```python
from build123d import *

# Parameters (mm, degrees)
SKETCH_W     = 15.4
SKETCH_H     = 6.2
SKETCH_R     = 1.6
PAD_DEPTH    = 6.2
SKETCH001_R  = 1.6
POCKET_DEPTH = 6.201
FILLET_R     = 3
FILLET001_R  = 3


with BuildPart() as part:
    # Sketch → Pad (new body)
    with BuildSketch(Plane.XY):
        with Locations((4.6, 0)):
            Rectangle(SKETCH_W, SKETCH_H)
        Circle(SKETCH_R, mode=Mode.SUBTRACT)
    extrude(amount=PAD_DEPTH)

    # Sketch001 (on Face1 of Pad) → Pocket (cut, through all)
    with BuildSketch(Plane(origin=(0, 3.1, 0), x_dir=(-1, 0, 0), z_dir=(0, 1, 0))):
        with Locations((-9.2, 3.1)):
            Circle(SKETCH001_R)
    extrude(amount=-POCKET_DEPTH, mode=Mode.SUBTRACT)

    # Fillet
    fillet_edges = [part.edges().sort_by_distance(p)[0] for p in [
        (-3.1, -3.1, 3.1),
        (-3.1, 3.1, 3.1),
    ]]
    fillet(fillet_edges, radius=FILLET_R)

    # Fillet001
    fillet001_edges = [part.edges().sort_by_distance(p)[0] for p in [
        (12.3, 0, 6.2),
        (12.3, 0, 0),
    ]]
    fillet(fillet001_edges, radius=FILLET001_R)


solid = part.part
```
CAD build for the part. Positions are in the model's coordinates, mm. Coordinates: 2 decimals unless noted, no trailing zeros. Order: outer loops, then holes, each group sorted by start corner. A loop starts at its lowest first (then second) coordinate and runs counter-clockwise, first axis right, second up. Notation, with made-up numbers: (34, 79) -> (64, 79) arc R14 ccw to (64, 89) -> close; hole circle Ø2 at (32, 69). An arc over 180 degrees is marked (long way). Use one line per item in the form item = value. Start each with the question number.
1) Pull direction Y, two halves, no side cores. Call faces 1 (the cylindrical face through (-2.24, -2.2, 3.14)), 2 (the cylindrical face through (-1.27, -0.97, 3.06)), 3 (the flat face through (4, 0, 6.2)), 4 (the cylindrical face through (-2.24, 2.2, 3.14)): +Y half, -Y half, draft (parallel to the pull), parting line (faces both ways), or undercut.
2) Drill centre lines: L1, parallel to X at y = 0.5, z = 2.25; L2, parallel to Z at x = 9.2, y = 1.5; L3, parallel to X at y = 0.5, z = 4.25. Where is each one in solid material? Low to high. Write a range as [from, to].
3) Drop a flat-ended pin along its axis: pin 1 (2 mm diameter, centred on y = -1, z = 5, fed in from -X). Give the stop position or say it passes through.
4) Band-saw the part on B-B on z = 2.75. Give the cut face in (x, y), then the cut area to 3 significant figures.
5) Band-saw the part on D-D on z = 5.75. Give the cut face in (x, y), then the cut area to 3 significant figures.
6) Band-saw the part on A-A on y = 1.25. Give the cut face in (x, z).
7) Band-saw the part on C-C on x = 0.25. Give the cut face in (y, z), then the cut area to 3 significant figures.
Entries:
q1.face_1 = -Y half
q1.face_2 = undercut
q1.face_3 = draft
q1.face_4 = +Y half
q2.L1 = [-3.07, -1.52], [1.52, 7.84], [10.56, 12.2]
q2.L2 = [0, 1.5], [4.7, 6.2]
q2.L3 = [-3.07, -1.52], [1.52, 8.09], [10.31, 12.11]
q3.pin_1 = -3.1
q4.outline = (-3.1, -0.1) arc R3 ccw to (-0.1, -3.1) -> (7.64, -3.1) -> (7.64, 3.1) -> (-0.1, 3.1) arc R3 ccw to (-3.1, 0.1) -> close; (10.76, -3.1) -> (12.29, -3.1) -> (12.29, 3.1) -> (10.76, 3.1) -> close; hole circle Ø3.2 at (0, 0)
q4.area = 64.2 mm2
q5.outline = (-3.1, -0.1) arc R3 ccw to (-0.1, -3.1) -> (10.88, -3.1) -> (10.88, 3.1) -> (-0.1, 3.1) arc R3 ccw to (-3.1, 0.1) -> close; hole circle Ø3.2 at (0, 0)
q5.area = 74.8 mm2
q6.outline = (-2.87, 0) -> (-1, 0) -> (-1, 6.2) -> (-2.87, 6.2) -> close; (1, 0) -> (9.3, 0) arc R3 ccw to (12.3, 3) -> (12.3, 3.2) arc R3 ccw to (9.3, 6.2) -> (1, 6.2) -> close; hole circle Ø3.2 at (9.2, 3.1)
q7.outline = (-3.1, 0) -> (-1.58, 0) -> (-1.58, 6.2) -> (-3.1, 6.2) -> close; (1.58, 0) -> (3.1, 0) -> (3.1, 6.2) -> (1.58, 6.2) -> close
q7.area = 18.8 mm2
